Part print with two shaded views. Sizes in mm from the minimum x, y, z corner. A direction names the side the tool comes from. Give positions to 0.01 mm unless a question says otherwise; leave off trailing zeros. Write each loop counter-clockwise with the first axis right and the second up, starting at its lowest first coordinate (ties: lowest second). Pieces come first, ordered by that corner, then holes. Notation, with made-up numbers: (-3, -29.75) - (32, -29.75) arc R12 ccw to (32, -24.75) - close; hole circle Ø5 at (89, 15). An arc over 180 degrees is marked (long way). One line per item, written item: value. Start each with the question number.
(1) Cut at B-B, the plane x = 5. List the corners of the cut face in (y, z), and give its area (4 significant figures).
(2) Probe L1, parallel to X at y = 4.5, z = 7; L2, parallel to X at y = 2, z = 5; L3, parallel to Z at x = 6.5, y = 4. List the from-to ranges inside material, lowest first.
(3) 3-axis set-ups, long thin cutter, end or side, ignore diameter. For the marked faces 1 and 2: which of +Z, -Z, +X, -X, +Y, -Y reach the whole face in a straight line?
(4) Drop flat-ended pins along their axis: P1, Ø3, axis at x = 9, z = 6, coming from the -Y side; P2, Ø0.5, axis at x = 5.5, y = 8.5, coming from the +Z side; P3, Ø1.9, axis at x = 5, y = 8.5, coming from the -Z side. Give the stop position or say it passes through.
(5) Cut at C-C, the plane y = 1.25. List the corners of the cut face in (x, z).
(6) Cut at A-A, the plane y = 8. List the corners of the cut face in (x, z), and give its area (3 significant figures).
(7) Mould opens along Z. For the marked faces 3, 4 and 5 say: pulls with the +Z half, pulls with the -Z half, needs draft (parallel to the pull), parting line crosses it, or undercut.
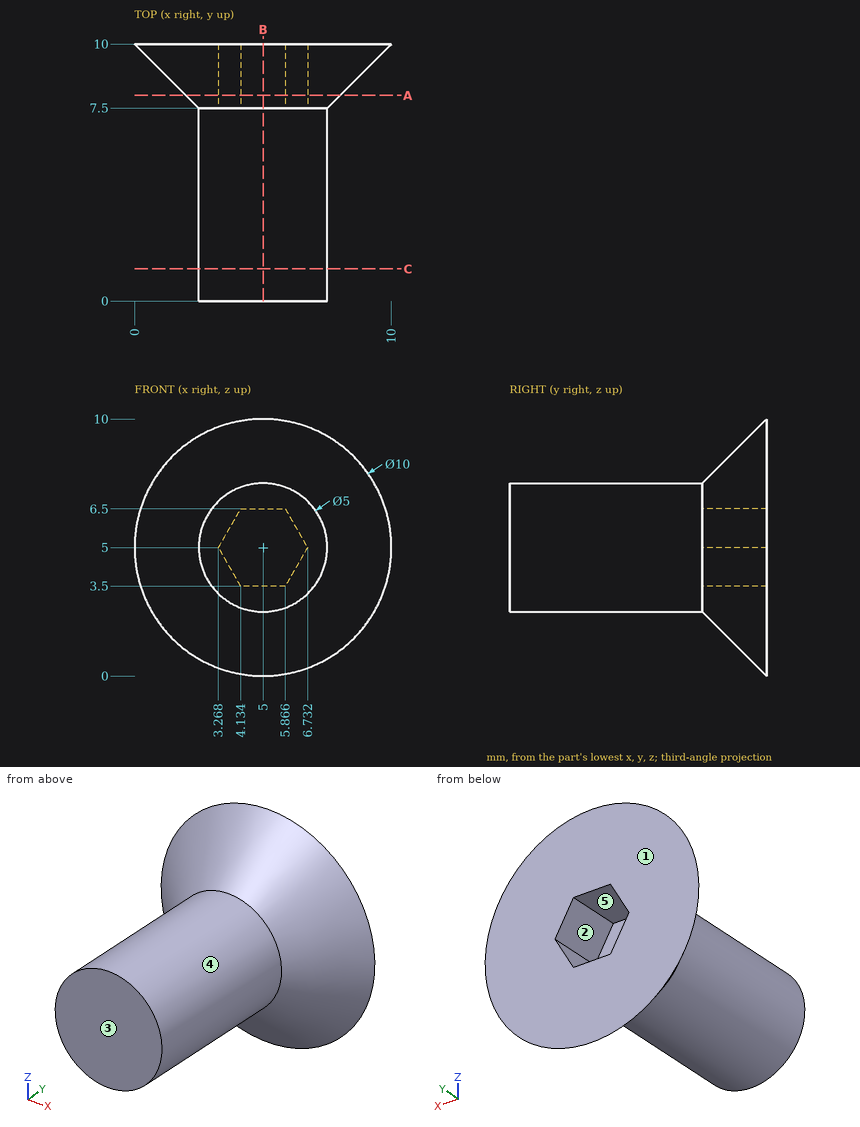
Answers follow:
1. outline: (0, 2.5) - (7.5, 2.5) - (10, 0) - (10, 3.5) - (7.5, 3.5) - (7.5, 6.5) - (10, 6.5) - (10, 10) - (7.5, 7.5) - (0, 7.5) - close
1. area: 48.75 mm²
2. L1: x = 3.5 to 6.5
2. L2: x = 2.5 to 7.5
2. L3: z = 3 to 7
3. face 1: +Z, -Z, +X, -X, +Y
3. face 2: +Y
4. P1: stops at y = 7.62
4. P2: stops at z = 8.72
4. P3: stops at z = 0.55
5. outline: circle Ø5 at (5, 5)
6. outline: circle Ø6 at (5, 5); hole (3.27, 5) - (4.13, 3.5) - (5.87, 3.5) - (6.73, 5) - (5.87, 6.5) - (4.13, 6.5) - close
6. area: 20.5 mm²
7. face 3: needs draft
7. face 4: parting line crosses it
7. face 5: undercut
